Geometry: final body of the model. Coordinates: model frame, mm. A direction names the side the tool comes from. Round coordinates to 2 decimals unless told otherwise and drop trailing zeros. Loops run counter-clockwise (first coordinate to the right, second up) from the corner with the lowest first, then second, coordinate; pieces in that order, holes last. Notation, with made-up numbers: (30, 9.25) - (34, 9.25) arc R17 cw to (34, 41.25) - close; hole circle Ø7 at (15, 31). An arc over 180 degrees is marked (long way). Use CSV: the item, a comma, the result in double quotes.
from build123d import *

# Parameters (mm, degrees)
SKETCH1_W           = 81.56143141
SKETCH1_H           = 54.816869018
BOSS_EXTRUDE1_DEPTH = 90
SKETCH2_W           = 10.019793311
SKETCH2_H           = 40.301038966


with BuildPart() as part:
    # Sketch1 → Boss-Extrude1 (new body)
    with BuildSketch(Plane(origin=(-20.318735881, -25.313413314, 0), x_dir=(1, 0, 0), z_dir=(0, 0, 1))):
        with Locations((14.605186555, -6.069687919)):
            Rectangle(SKETCH1_W, SKETCH1_H)
    extrude(amount=BOSS_EXTRUDE1_DEPTH)

    # Sweep3: sweep along a path in Sketch3
    with BuildLine(Plane(origin=(0, -10.087901928, 0), x_dir=(1, 0, 0), z_dir=(0, 1, 0))) as sweep3_path:
        Line((35.067166378, -76.74628409), (89.647981196, -76.74628409))
        Line((89.647981196, -76.74628409), (89.647981196, -11.63207723))
        Line((89.647981196, -11.63207723), (35.067166378, -11.63207723))
    # Sketch2 → Sweep3 (sweep)
    with BuildSketch(Plane(origin=(35.067166378, 0, 0), x_dir=(0, 0, -1), z_dir=(1, 0, 0))):
        with Locations((-76.74628409, -30.238421411)):
            Rectangle(SKETCH2_W, SKETCH2_H)
    sweep(path=sweep3_path.line, transition=Transition.RIGHT)


solid = part.part
Item 1: Reachability of faces 1 (the flat face through (65, -30, 81.756)), 2 (the flat face through (84.638, -31, 44)), 3 (the flat face through (85, -10.088, 44)), 4 (the flat face through (85, -50.389, 45)), 5 (the flat face through (64, -30, 6.622)) from +Z, -Z, +X, -X, +Y, -Y: full face, straight path, thin tool, end or side. Return the list, or none.
Final values:
face 1,"+Z, +X, +Y, -Y"
face 2,"+Y, -Y"
face 3,"+Z, -Z, +X, +Y"
face 4,"+Z, -Z, +X, -Y"
face 5,"-Z, +X, +Y, -Y"
Item 2: Mould query, pull axis X, two halves, no side actions, for faces 6 (the flat face through (-6, -31, 90)), 7 (the flat face through (60, -31, 71.736)), 8 (the flat face through (94.658, -30, 44)), 9 (the flat face through (60, -31, 16.642)). Classes: released by +X, released by -X, zero draft, split by the parting line, or undercut.
Final values:
face 6,"zero draft"
face 7,"undercut"
face 8,"released by +X"
face 9,"undercut"
Item 3: Section D-D on z = 79.5. Return the cut outline in (x, y).
Final values:
outline,"(-46.49, -58.79) - (35.07, -58.79) - (35.07, -50.39) - (94.66, -50.39) - (94.66, -10.09) - (35.07, -10.09) - (35.07, -3.97) - (-46.49, -3.97) - close"
Item 4: Material intervals for line 1 (X direction, y = -25, z = 46); line 2 (Z direction, x = 60.5, y = -13.5); line 3 (Y direction, x = 76, z = 12.5), sorted ascending.
Final values:
line 1,"x = -46.49 to 35.07, 84.64 to 94.66"
line 2,"z = 6.62 to 16.64, 71.74 to 81.76"
line 3,"y = -50.39 to -10.09"
Item 5: Section A-A on x = 47. Return the cut outline in (y, z).
Final values:
outline,"(-50.39, 6.62) - (-10.09, 6.62) - (-10.09, 16.64) - (-50.39, 16.64) - close; (-50.39, 71.74) - (-10.09, 71.74) - (-10.09, 81.76) - (-50.39, 81.76) - close"
Item 6: Pin query (flat end, axial travel): P1, Ø4, axis at x = 69, y = -50, coming from the +Z side; P2, Ø12, axis at x = 56.5, y = -34.5, coming from the -Z side; P3, Ø18, axis at x = 61.5, z = 60, coming from the +Y side. Return the tip coordinate at first contact, or that it passes through.
Final values:
P1,"stops at z = 81.76"
P2,"stops at z = 6.62"
P3,"passes through"
Item 7: Section B-B on y = -14.5. Return the cut outline in (x, z).
Final values:
outline,"(-46.49, 0) - (35.07, 0) - (35.07, 6.62) - (94.66, 6.62) - (94.66, 81.76) - (35.07, 81.76) - (35.07, 90) - (-46.49, 90) - close; hole (35.07, 16.64) - (84.64, 16.64) - (84.64, 71.74) - (35.07, 71.74) - close"
Item 8: Section C-C on z = 24. Return the cut outline in (x, y).
Final values:
outline,"(-46.49, -58.79) - (35.07, -58.79) - (35.07, -3.97) - (-46.49, -3.97) - close; (84.64, -50.39) - (94.66, -50.39) - (94.66, -10.09) - (84.64, -10.09) - close"
